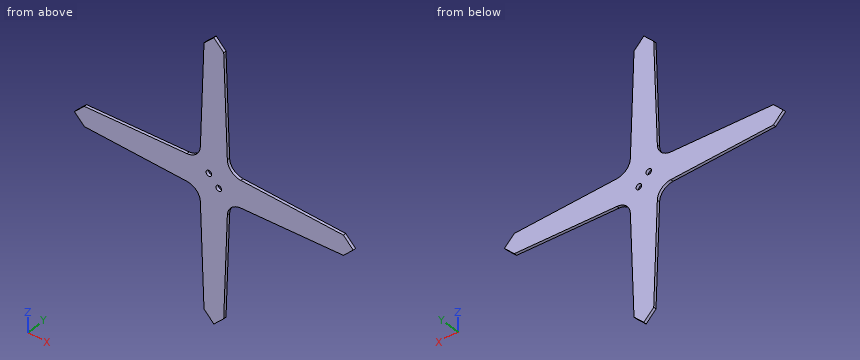
```python
from build123d import *

# Parameters (mm, degrees)
SKETCH1_R           = 3
BOSS_EXTRUDE1_DEPTH = 3
FILLET1_R           = 15


with BuildPart() as part:
    # Sketch1 → Boss-Extrude1 (new body)
    with BuildSketch(Plane(origin=(0, 0, 0), x_dir=(1, 0, 0), z_dir=(0, 1, 0))):
        Polygon((-286.26, 15), (-410.653398282, 10.606601718), (-421.26, 0), (-410.653398282, -10.606601718), (-286.26, -15), (-281.866601718, -139.393398282), (-271.26, -150), (-260.653398282, -139.393398282), (-256.26, -15), (-131.866601718, -10.606601718), (-121.26, 0), (-131.866601718, 10.606601718), (-256.26, 15), (-260.653398282, 139.393398282), (-271.26, 150), (-281.866601718, 139.393398282), align=None)
        with Locations(Location((-276.563300859, -5.303300859, 0), (0, 0, 270))):
            Circle(SKETCH1_R, mode=Mode.SUBTRACT)
        with Locations(Location((-265.956699141, 5.303300859, 0), (0, 0, 270))):
            Circle(SKETCH1_R, mode=Mode.SUBTRACT)
    extrude(amount=BOSS_EXTRUDE1_DEPTH)

    # Fillet1
    fillet1_edges = [part.edges().sort_by_distance(p)[0] for p in [
        (-256.26, 1.5, -15),
        (-256.26, 1.5, 15),
        (-286.26, 1.5, 15),
        (-286.26, 1.5, -15),
    ]]
    fillet(fillet1_edges, radius=FILLET1_R)


solid = part.part
```
Verification items for the finished model (mm, model axes). Coordinates: 2 decimals unless noted, no trailing zeros. Order: outer loops, then holes, each group sorted by start corner. A loop starts at its lowest first (then second) coordinate and runs counter-clockwise, first axis right, second up. Notation, with made-up numbers: (-25.75, 82) -> (-14.75, 82) arc R19 ccw to (-14.75, 110) -> close; hole circle Ø4 at (-18.5, 15). An arc over 180 degrees is marked (long way). Put each result on its own line as item: value. Start each with the question number.
1) Cross-section at C-C (z = -108). Enter the section's corners in (x, y).
2) Go/stop test with flat-tipped pins: pin 1 (1 mm diameter, centred on x = -275.5, y = 2, fed in from +Z); pin 2 (1.5 mm diameter, centred on x = -349, y = 2.5, fed in from -Z); pin 3 (1.5 mm diameter, centred on x = -223, y = 0.5, fed in from +Z). Record where each tip stops, or that it passes through.
3) Material ranges on L1, parallel to X at y = 2, z = -6; L2, parallel to X at y = 2.8, z = 6; L3, parallel to Z at x = -266, y = 1.6, recorded low to high.
4) Cross-section at B-B (x = -350). Enter the section's corners in (y, z).
5) Cross-section at A-A (y = 2). Enter the section's corners in (x, z).
Geometry check:
1. outline: (-282.98, 0) -> (-259.54, 0) -> (-259.54, 3) -> (-282.98, 3) -> close
2. pin 1: stops at z = 146.26
2. pin 2: stops at z = -12.81
2. pin 3: stops at z = 13.85
3. L1: x = -415.26 to -268.87, -263.04 to -127.26
3. L2: x = -415.26 to -279.48, -273.65 to -127.26
3. L3: z = -144.74 to -8.3, -2.3 to 144.74
4. outline: (0, -12.75) -> (3, -12.75) -> (3, 12.75) -> (0, 12.75) -> close
5. outline: (-421.26, 0) -> (-410.65, -10.61) -> (-300.23, -14.51) arc R15 cw to (-285.77, -28.97) -> (-281.87, -139.39) -> (-271.26, -150) -> (-260.65, -139.39) -> (-256.75, -28.97) arc R15 cw to (-242.29, -14.51) -> (-131.87, -10.61) -> (-121.26, 0) -> (-131.87, 10.61) -> (-242.29, 14.51) arc R15 cw to (-256.75, 28.97) -> (-260.65, 139.39) -> (-271.26, 150) -> (-281.87, 139.39) -> (-285.77, 28.97) arc R15 cw to (-300.23, 14.51) -> (-410.65, 10.61) -> close; hole circle Ø6 at (-276.56, 5.3); hole circle Ø6 at (-265.96, -5.3)
